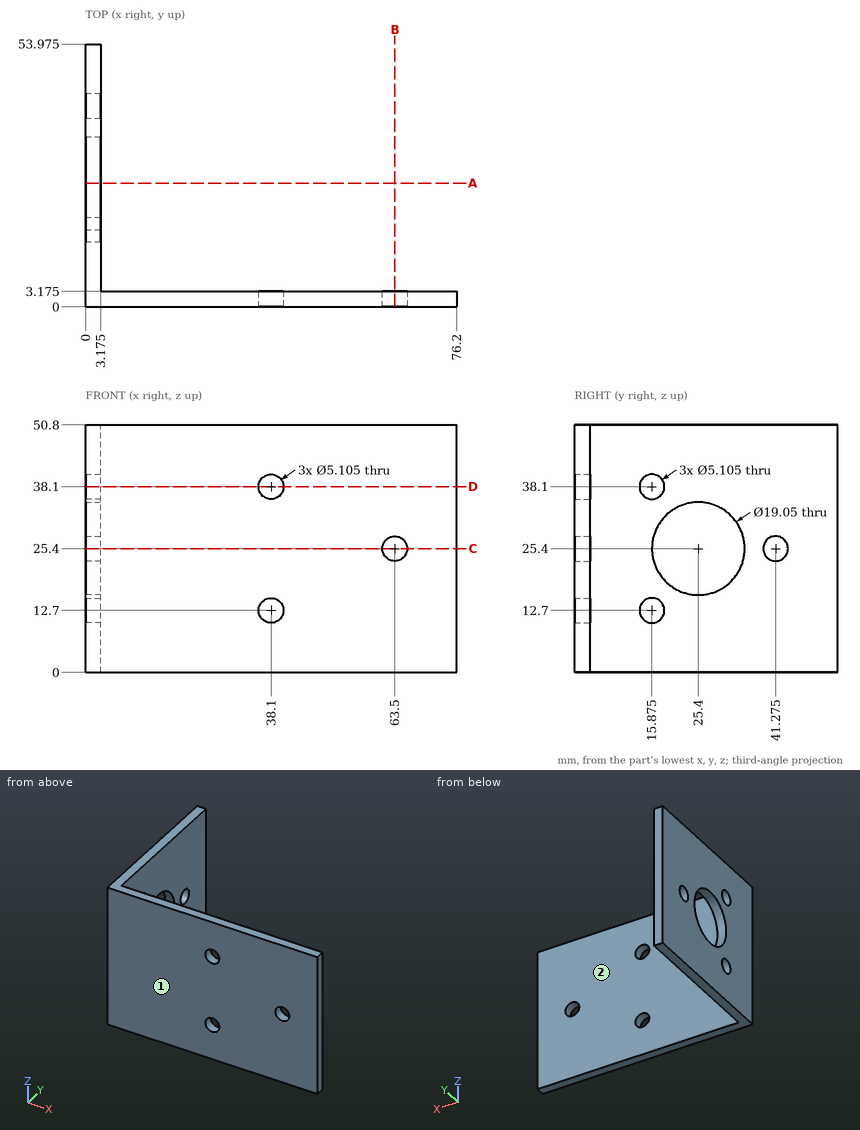
Verification items for this drawing (mm, ordinates from the low corner). A direction names the side the tool comes from. Round coordinates to 2 decimals unless told otherwise and drop trailing zeros. Order: outer loops, then holes, each group sorted by start corner. A loop starts at its lowest first (then second) coordinate and runs counter-clockwise, first axis right, second up. Notation, with made-up numbers: (80.25, 7) - (92.25, 7) arc R17 cw to (92.25, 19) - close; hole circle Ø9 at (4.5, 11.25). An arc over 180 degrees is marked (long way). Answer as CSV lines item,"result". Start each with the question number.
1) Scan lines: probe 1 along Y at (x, z) = (2.2, 25.4) (1 decimal); probe 2 along Y at (x, z) = (2.05, 12.7) (1 decimal); probe 3 along X at (y, z) = (0.85, 25.4). Record each from-to range of solid material in increasing order.
2) Section check B-B (x = 63.5). Record the cut outline in (y, z) (1 decimal).
3) Section check C-C (z = 25.4). Record the cut outline in (x, y) (1 decimal), then the cut area to 3 significant figures.
4) Depth check by flat-ended pin: pin 1 (17 mm diameter, centred on y = 25.4, z = 25.4, fed in from +X); pin 2 (1 mm diameter, centred on y = 9, z = 7.5, fed in from +X) (3 decimals); pin 3 (3 mm diameter, centred on x = 56, z = 34.5, fed in from +Y) (3 decimals). Enter the tip coordinate at first touch or a pass-through.
5) Section check A-A (y = 25.4). Record the cut outline in (x, z) (1 decimal), then the cut area to 3 significant figures.
6) Section check D-D (z = 38.1). Record the cut outline in (x, y) (1 decimal).
7) Tool access check on the marked faces 1 and 2. Record the directions out of +Z, -Z, +X, -X, +Y, -Y that give a thin tool (end or side, any length) a straight path to the whole face; none if there is none.
Determined:
1,probe 1,"0 to 15.9, 34.9 to 38.7, 43.8 to 54"
1,probe 2,"0 to 13.3, 18.4 to 54"
1,probe 3,"0 to 60.95, 66.05 to 76.2"
2,outline,"(0, 0) - (3.2, 0) - (3.2, 22.8) - (0, 22.8) - close; (0, 28) - (3.2, 28) - (3.2, 50.8) - (0, 50.8) - close"
3,outline,"(0, 0) - (60.9, 0) - (60.9, 3.2) - (3.2, 3.2) - (3.2, 15.9) - (0, 15.9) - close; (0, 34.9) - (3.2, 34.9) - (3.2, 38.7) - (0, 38.7) - close; (0, 43.8) - (3.2, 43.8) - (3.2, 54) - (0, 54) - close; (66.1, 0) - (76.2, 0) - (76.2, 3.2) - (66.1, 3.2) - close"
3,area,"310 mm^2"
4,pin 1,"through"
4,pin 2,"x = 3.175"
4,pin 3,"y = 3.175"
5,outline,"(0, 0) - (3.2, 0) - (3.2, 15.9) - (0, 15.9) - close; (0, 34.9) - (3.2, 34.9) - (3.2, 50.8) - (0, 50.8) - close"
5,area,"101 mm^2"
6,outline,"(0, 0) - (35.5, 0) - (35.5, 3.2) - (3.2, 3.2) - (3.2, 13.3) - (0, 13.3) - close; (0, 18.4) - (3.2, 18.4) - (3.2, 54) - (0, 54) - close; (40.7, 0) - (76.2, 0) - (76.2, 3.2) - (40.7, 3.2) - close"
7,face 1,"+Z, -Z, +X, -X, -Y"
7,face 2,"+Z, -Z, +X, +Y"
